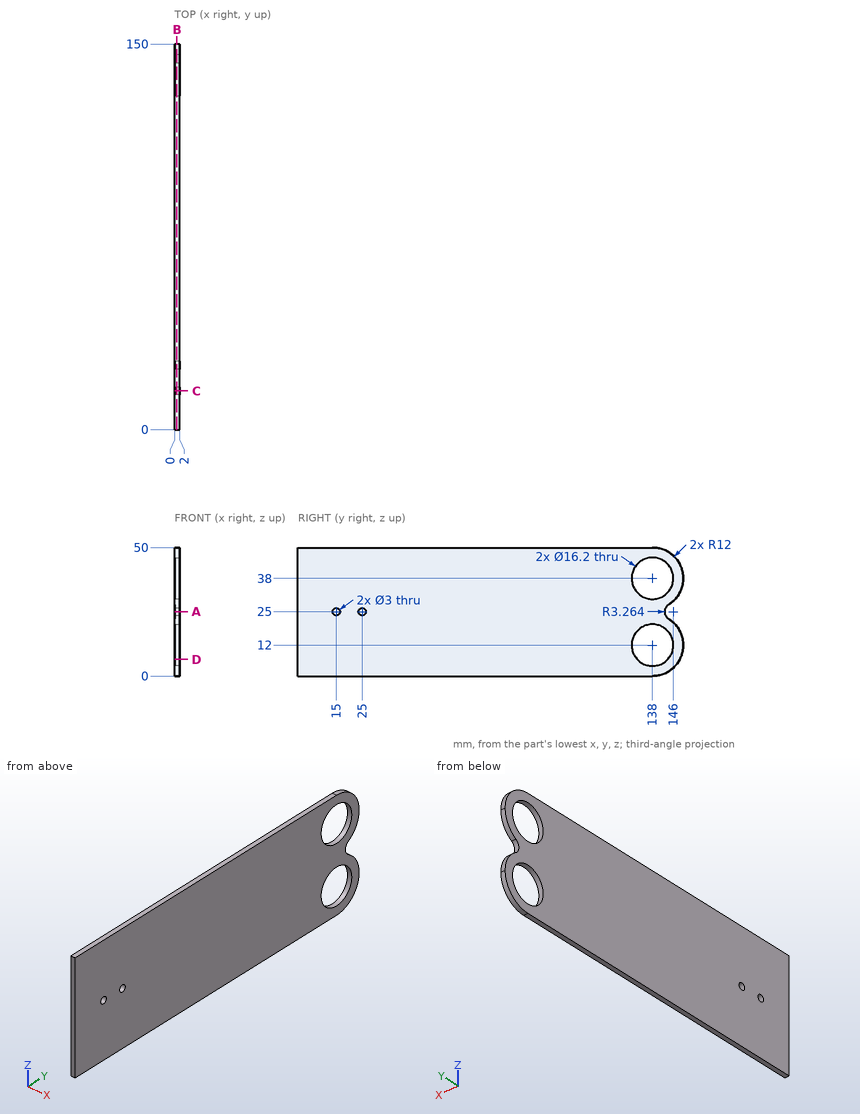
Geometry: see drawing. Coordinates: mm, zero at the bounding-box minimum. Give positions to 0.01 mm unless a question says otherwise; leave off trailing zeros. Loops run counter-clockwise (first coordinate to the right, second up) from the corner with the lowest first, then second, coordinate; pieces in that order, holes last. Notation, with made-up numbers: M 87.25,26.5 L 139.25,26.5 A10 ccw 139.25,45.5 Z; hole C -2.75,66 d10. An arc over 180 degrees is marked long. Answer as CSV lines item,"result". Start each with the question number.
1. Section C-C on y = 15. Return loops of the section in (x, z).
2. Line query: L1, parallel to Y at x = 0.75, z = 25 (1 decimal); L2, parallel to Z at x = 1.4, y = 25; L3, parallel to Y at x = 1.5, z = 12. Output: solid intervals per line, ascending.
3. Section B-B on x = 0.85. Return loops of the section in (y, z) (1 decimal).
4. Section D-D on z = 6.5. Return loops of the section in (x, y) (1 decimal).
5. Section A-A on z = 25. Return loops of the section in (x, y) (1 decimal).
Computed values:
1,outline,"M 0,0 L 2,0 L 2,23.5 L 0,23.5 Z; M 0,26.5 L 2,26.5 L 2,50 L 0,50 Z"
2,L1,"y = 0 to 13.5, 16.5 to 23.5, 26.5 to 142.7"
2,L2,"z = 0 to 23.5, 26.5 to 50"
2,L3,"y = 0 to 129.9, 146.1 to 150"
3,outline,"M 0,0 L 138,0 A12 ccw 144.3,22.2 A3.3 cw 144.3,27.8 A12 ccw 138,50 L 0,50 Z; hole C 15,25 d3; hole C 25,25 d3; hole C 138,12 d16.2; hole C 138,38 d16.2"
4,outline,"M 0,0 L 2,0 L 2,132.1 L 0,132.1 Z; M 0,143.9 L 2,143.9 L 2,148.7 L 0,148.7 Z"
5,outline,"M 0,0 L 2,0 L 2,13.5 L 0,13.5 Z; M 0,16.5 L 2,16.5 L 2,23.5 L 0,23.5 Z; M 0,26.5 L 2,26.5 L 2,142.7 L 0,142.7 Z"
